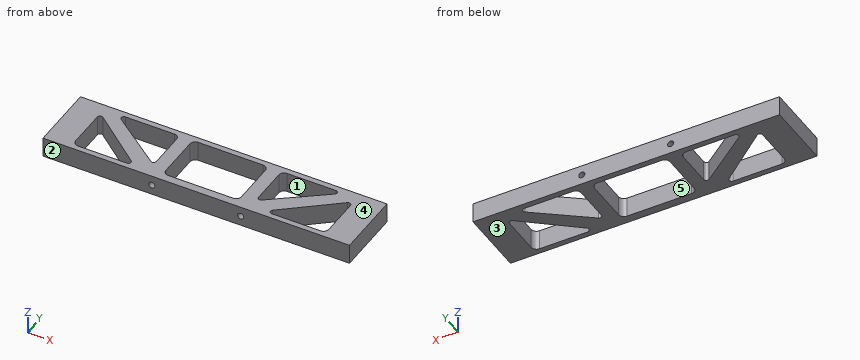
from build123d import *

# Parameters (mm, degrees)
BOSS_EXTRUDE2_DEPTH                        = 9.525
SKETCH4_R                                  = 1.4732
CUT_EXTRUDE2_DEPTH                         = 12.7
MIRROR2_AT_THE_SECOND_PLANE_COPY_1_SKETC_R = 1.4732
MIRROR2_AT_THE_SECOND_PLANE_COPY_1_DEPTH   = 12.7


with BuildPart() as part:
    # Sketch2 → Boss-Extrude2 (new body)
    with BuildSketch(Plane.XY):
        Polygon((-63.5, 15.299999878), (-73.025, 15.299999878), (-73.025, -16.450000122), (-63.5, -16.450000122), (-21.166666667, -16.450000122), (0, -16.450000122), (73.025, -16.450000122), (73.025, 15.299999878), (-21.166666667, 15.299999878), (-24.341666667, 15.299999878), align=None)
        with BuildLine():
            ThreePointArc((-57.785, -13.912500244), (-59.581051224, -13.168551468), (-60.325, -11.372500244))
            Line((-60.325, -11.372500244), (-60.325, 6.985))
            ThreePointArc((-60.325, 6.985), (-59.605365306, 8.129551454), (-58.262010976, 7.977002221))
            Line((-58.262010976, 7.977002221), (-33.708677642, -11.650498023))
            ThreePointArc((-33.708677642, -11.650498023), (-33.303179533, -13.062653299), (-34.501666667, -13.912500244))
            Line((-34.501666667, -13.912500244), (-57.785, -13.912500244))
        make_face(mode=Mode.SUBTRACT)
        with BuildLine():
            ThreePointArc((60.325, -11.372500244), (59.581051224, -13.168551468), (57.785, -13.912500244))
            Line((57.785, -13.912500244), (34.501666667, -13.912500244))
            ThreePointArc((34.501666667, -13.912500244), (33.303179533, -13.062653299), (33.708677642, -11.650498023))
            Line((33.708677642, -11.650498023), (58.262010976, 7.977002221))
            ThreePointArc((58.262010976, 7.977002221), (59.605365306, 8.129551454), (60.325, 6.985))
            Line((60.325, 6.985), (60.325, -11.372500244))
        make_face(mode=Mode.SUBTRACT)
        with BuildLine():
            Line((-26.373666667, -8.001), (-50.927, 10.414))
            ThreePointArc((-50.927, 10.414), (-51.369827789, 11.831609263), (-50.165, 12.7))
            Line((-50.165, 12.7), (-26.881666667, 12.7))
            ThreePointArc((-26.881666667, 12.7), (-25.085615442, 11.956051224), (-24.341666667, 10.16))
            Line((-24.341666667, 10.16), (-24.341666667, -6.985))
            ThreePointArc((-24.341666667, -6.985), (-25.0437054, -8.120922533), (-26.373666667, -8.001))
        make_face(mode=Mode.SUBTRACT)
        with BuildLine():
            ThreePointArc((-17.991666667, 10.16), (-17.247717891, 11.956051224), (-15.451666667, 12.7))
            Line((-15.451666667, 12.7), (15.451666667, 12.7))
            ThreePointArc((15.451666667, 12.7), (17.247717891, 11.956051224), (17.991666667, 10.16))
            Line((17.991666667, 10.16), (17.991666667, -10.16))
            ThreePointArc((17.991666667, -10.16), (17.247717891, -11.956051224), (15.451666667, -12.7))
            Line((15.451666667, -12.7), (-15.451666667, -12.7))
            ThreePointArc((-15.451666667, -12.7), (-17.247717891, -11.956051224), (-17.991666667, -10.16))
            Line((-17.991666667, -10.16), (-17.991666667, 10.16))
        make_face(mode=Mode.SUBTRACT)
        with BuildLine():
            Line((24.341666667, -6.985), (24.341666667, 10.16))
            ThreePointArc((24.341666667, 10.16), (25.085615442, 11.956051224), (26.881666667, 12.7))
            Line((26.881666667, 12.7), (50.165, 12.7))
            ThreePointArc((50.165, 12.7), (51.369827789, 11.831609263), (50.927, 10.414))
            Line((50.927, 10.414), (26.373666667, -8.001))
            ThreePointArc((26.373666667, -8.001), (25.0437054, -8.120922533), (24.341666667, -6.985))
        make_face(mode=Mode.SUBTRACT)
    extrude(amount=BOSS_EXTRUDE2_DEPTH)

    # Sketch4 → Cut-Extrude2 (cut)
    with BuildSketch(Plane(origin=(0, 15.299999878, 0), x_dir=(1, 0, 0), z_dir=(0, 1, 0))):
        with Locations((21.166666667, -4.7625)):
            Circle(SKETCH4_R)
    cut_extrude2 = extrude(amount=-CUT_EXTRUDE2_DEPTH, mode=Mode.SUBTRACT)

    # Mirror2: Cut-Extrude2 across plane
    add(cut_extrude2.mirror(Plane.ZX.offset(-0.575000122)), mode=Mode.SUBTRACT)

    # Mirror2 at the second plane: Cut-Extrude2 across plane
    add(cut_extrude2.mirror(Plane(origin=(0, 0, 0), x_dir=(0, 0, 1), z_dir=(1, 0, 0))), mode=Mode.SUBTRACT)

    # Mirror2 at the second plane copy 1 sketc → Mirror2 at the second plane copy 1 (cut)
    with BuildSketch(Plane(origin=(0, -16.450000122, 0), x_dir=(-1, 0, 0), z_dir=(0, -1, 0))):
        with Locations((21.166666667, -4.7625)):
            Circle(MIRROR2_AT_THE_SECOND_PLANE_COPY_1_SKETC_R)
    extrude(amount=-MIRROR2_AT_THE_SECOND_PLANE_COPY_1_DEPTH, mode=Mode.SUBTRACT)


solid = part.part
Model file for the job. Use its own axes, mm. Face numbers are marked on the shaded views. A direction names the side the tool comes from. Give positions to 0.01 mm unless a question says otherwise; leave off trailing zeros. Write each loop counter-clockwise with the first axis right and the second up, starting at its lowest first coordinate (ties: lowest second). Pieces come first, ordered by that corner, then holes. Notation, with made-up numbers: (47.5, 23.5) -> (96.5, 23.5) arc R10 ccw to (96.5, 41.5) -> close; hole circle Ø5 at (15, 66). An arc over 180 degrees is marked (long way). Write item = value, one per line.
(1) Mould opens along Y. For the marked faces 1, 2 and 3 say: released by +Y, released by -Y, zero draft, split by the parting line, or undercut.
Determined:
face_1 = undercut
face_2 = released by -Y
face_3 = zero draft
(2) Tool access for the marked faces 4 and 5: list every direction of +Z, -Z, +X, -X, +Y, -Y with a clear straight run to the whole face (end or side of a thin tool).
Determined:
face_4 = +Z, +X, -X, +Y, -Y
face_5 = +Z, -Z
(3) Flat gauge pins, fed straight in: P1, Ø1.8, axis at x = 21.17, z = 4.76, coming from the +Y side; P2, Ø1.5, axis at x = 21.5, z = 4.5, coming from the -Y side. Where does each tip first touch, or does it go through?
Determined:
P1 = 2.6
P2 = -3.75
(4) Probe line 1 along Y through (x, z) = (15, 2.75); line 2 along X through (y, z) = (-11.5, 6.75) (3 decimals); line 3 along Y through (x, z) = (-40.5, 5). List the from-to ranges inside material, lowest first.
Determined:
line_1 = -16.45 to -12.7, 12.7 to 15.3
line_2 = -73.025 to -60.322, -33.897 to -17.609, 17.609 to 33.897, 60.322 to 73.025
line_3 = -16.45 to -13.91, -6.22 to 2.59, 12.7 to 15.3
(5) Slice it at A-A, the plane x = -7.5. Give the cut face in (y, z) (3 decimals).
Determined:
outline = (-16.45, 0) -> (-12.7, 0) -> (-12.7, 9.525) -> (-16.45, 9.525) -> close; (12.7, 0) -> (15.3, 0) -> (15.3, 9.525) -> (12.7, 9.525) -> close
(6) Slice it at B-B, the plane x = -39. Give the number of separate pieces and of enclosed holes in the cut face, then the cut area to 3 significant figures.
Determined:
separate_pieces = 3
enclosed_holes = 0
area = 134 mm2
